Study the drawing (mm; zero at the part's minimum x, y, z) and answer. Give positions to 0.01 mm unless a question says otherwise; leave off trailing zeros. Write each loop counter-clockwise with the first axis right and the second up, starting at its lowest first coordinate (ties: lowest second). Pieces come first, ordered by that corner, then holes. Notation, with made-up numbers: (9, 10.25) -> (58, 10.25) arc R13 ccw to (58, 24.25) -> close; hole circle Ø7 at (35.25, 10.25). An arc over 180 degrees is marked (long way). One line per question, with ' | ' between items.
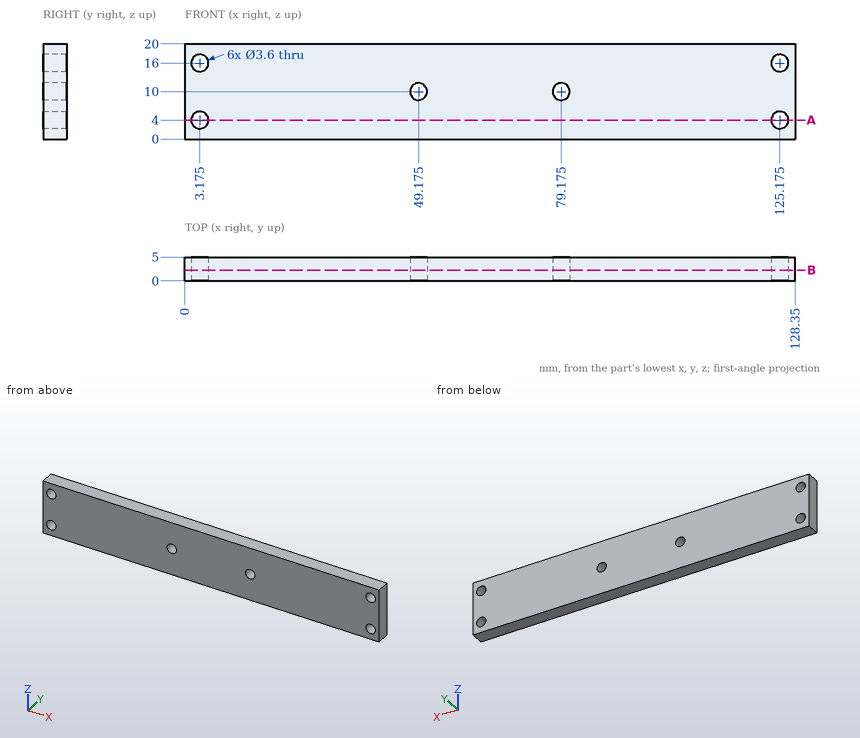
Item 1: Find section B-B (y = 2.25). Write down the section's boundary in (x, z) (3 decimals), then the cut area to 3 significant figures.
Answers below:
outline: (0, 0) -> (128.35, 0) -> (128.35, 20) -> (0, 20) -> close; hole circle Ø3.6 at (3.175, 4); hole circle Ø3.6 at (3.175, 16); hole circle Ø3.6 at (49.175, 10); hole circle Ø3.6 at (79.175, 10); hole circle Ø3.6 at (125.175, 4); hole circle Ø3.6 at (125.175, 16) | area: 2,510 mm²
Item 2: Consider line 1 (X direction, y = 3.65, z = 4) (3 decimals); line 2 (X direction, y = 1.4, z = 10) (3 decimals). Determine where each line is inside the solid, lowest interval first. Write a range as [from, to].
Answers below:
line 1: [0, 1.375], [4.975, 123.375], [126.975, 128.35] | line 2: [0, 47.375], [50.975, 77.375], [80.975, 128.35]
Item 3: Find section A-A (z = 4). Write down the section's boundary in (x, y) (3 decimals).
Answers below:
outline: (0, 0) -> (1.375, 0) -> (1.375, 5) -> (0, 5) -> close; (4.975, 0) -> (123.375, 0) -> (123.375, 5) -> (4.975, 5) -> close; (126.975, 0) -> (128.35, 0) -> (128.35, 5) -> (126.975, 5) -> close
